```python
from build123d import *

# Parameters (mm, degrees)
EXTRUDE_1_DEPTH     = 10
SKETCH_2_R          = 30
CUT_EXTRUDE_1_DEPTH = 10


with BuildPart() as part:
    # 草图1 → 凸台-拉伸1 (new body)
    with BuildSketch(Plane.XY):
        with BuildLine():
            Line((-24.04163056, 28.284271247), (-25.420200489, 29.906118222))
            ThreePointArc((-25.420200489, 29.906118222), (0, 39.25), (25.420200489, 29.906118222))
            Line((25.420200489, 29.906118222), (24.04163056, 28.284271247))
            ThreePointArc((24.04163056, 28.284271247), (24.04163056, 24.04163056), (28.284271247, 24.04163056))
            Line((28.284271247, 24.04163056), (29.906118222, 25.420200489))
            ThreePointArc((29.906118222, 25.420200489), (39.25, 0), (29.906118222, -25.420200489))
            Line((29.906118222, -25.420200489), (28.284271247, -24.04163056))
            ThreePointArc((28.284271247, -24.04163056), (24.04163056, -24.04163056), (24.04163056, -28.284271247))
            Line((24.04163056, -28.284271247), (25.420200489, -29.906118222))
            ThreePointArc((25.420200489, -29.906118222), (0, -39.25), (-25.420200489, -29.906118222))
            Line((-25.420200489, -29.906118222), (-24.04163056, -28.284271247))
            ThreePointArc((-24.04163056, -28.284271247), (-24.04163056, -24.04163056), (-28.284271247, -24.04163056))
            Line((-28.284271247, -24.04163056), (-29.906118222, -25.420200489))
            ThreePointArc((-29.906118222, -25.420200489), (-39.25, 0), (-29.906118222, 25.420200489))
            Line((-29.906118222, 25.420200489), (-28.284271247, 24.04163056))
            ThreePointArc((-28.284271247, 24.04163056), (-24.04163056, 24.04163056), (-24.04163056, 28.284271247))
        make_face()
    extrude(amount=EXTRUDE_1_DEPTH)

    # 草图2 → 切除-拉伸1 (cut)
    with BuildSketch(Plane(origin=(0, 0, 0), x_dir=(-1, 0, 0), z_dir=(0, 0, -1))):
        Circle(SKETCH_2_R)
    extrude(amount=-CUT_EXTRUDE_1_DEPTH, mode=Mode.SUBTRACT)


solid = part.part
```
Design review of the part built by this model. Coordinates are the model's own, in mm. Give positions to 0.01 mm unless a question says otherwise; leave off trailing zeros. Order: outer loops, then holes, each group sorted by start corner. A loop starts at its lowest first (then second) coordinate and runs counter-clockwise, first axis right, second up. Notation, with made-up numbers: (35.25, -37.75) -> (81.25, -37.75) arc R35 cw to (81.25, -0.75) -> close; hole circle Ø11 at (62, -13.75). An arc over 180 degrees is marked (long way). Write item = value, one per line. Start each with the question number.
(1) We need section C-C on z = 3.25. Write out the cut boundary in (x, y), plus the area to 3 significant figures.
(2) We need section A-A on x = 0. Write out the cut boundary in (y, z).
(3) To check wall thickness, follow line 1 along Y through (x, z) = (0, 7.5); line 2 along Y through (x, z) = (23.5, 9); line 3 along Y through (x, z) = (25, 5). State the ranges of each line that lie inside material, in increasing order.
(4) For pin 1 (2 mm diameter, centred on x = -7, z = 3.5, fed in from -Y); pin 2 (5 mm diameter, centred on x = -22.5, z = 4.5, fed in from +Y); pin 3 (6 mm diameter, centred on x = 10, z = 5, fed in from -Y), all flat-tipped, find the tip position at first contact; note any pin that passes through.
(5) Mouldability with a two-part tool opening along Y and no side actions: class faces 1 (the face through (29, -9, 10)), 2 (the face through (0.39, -39.25, 4.93)), 3 (the face through (29.97, 1.32, 4.93)), 4 (the face through (24.089, -23.995, 4.93)) as +Y half, -Y half, draft (parallel to the pull), parting line (faces both ways), or undercut.
Numbers:
q1.outline = (-29.91, -25.42) -> (-28.28, -24.04) arc R3 cw to (-24.04, -28.28) -> (-25.42, -29.91) arc R39.25 ccw to (25.42, -29.91) -> (24.04, -28.28) arc R3 cw to (28.28, -24.04) -> (29.91, -25.42) arc R39.25 ccw to (29.91, 25.42) -> (28.28, 24.04) arc R3 cw to (24.04, 28.28) -> (25.42, 29.91) arc R39.25 ccw to (-25.42, 29.91) -> (-24.04, 28.28) arc R3 cw to (-28.28, 24.04) -> (-29.91, 25.42) arc R39.25 ccw to start; hole circle Ø60 at (0, 0)
q1.area = 1,900 mm^2
q2.outline = (-39.25, 0) -> (-30, 0) -> (-30, 10) -> (-39.25, 10) -> close; (30, 0) -> (39.25, 0) -> (39.25, 10) -> (30, 10) -> close
q3.line_1 = -39.25 to -30, 30 to 39.25
q3.line_2 = -31.44 to -27.54, -24.78 to -18.65, 18.65 to 24.78, 27.54 to 31.44
q3.line_3 = -30.26 to -29.41, -23.4 to -16.58, 16.58 to 23.4, 29.41 to 30.26
q4.pin_1 = -38.79
q4.pin_2 = 33.77
q4.pin_3 = -38.62
q5.face_1 = draft
q5.face_2 = -Y half
q5.face_3 = undercut
q5.face_4 = undercut
